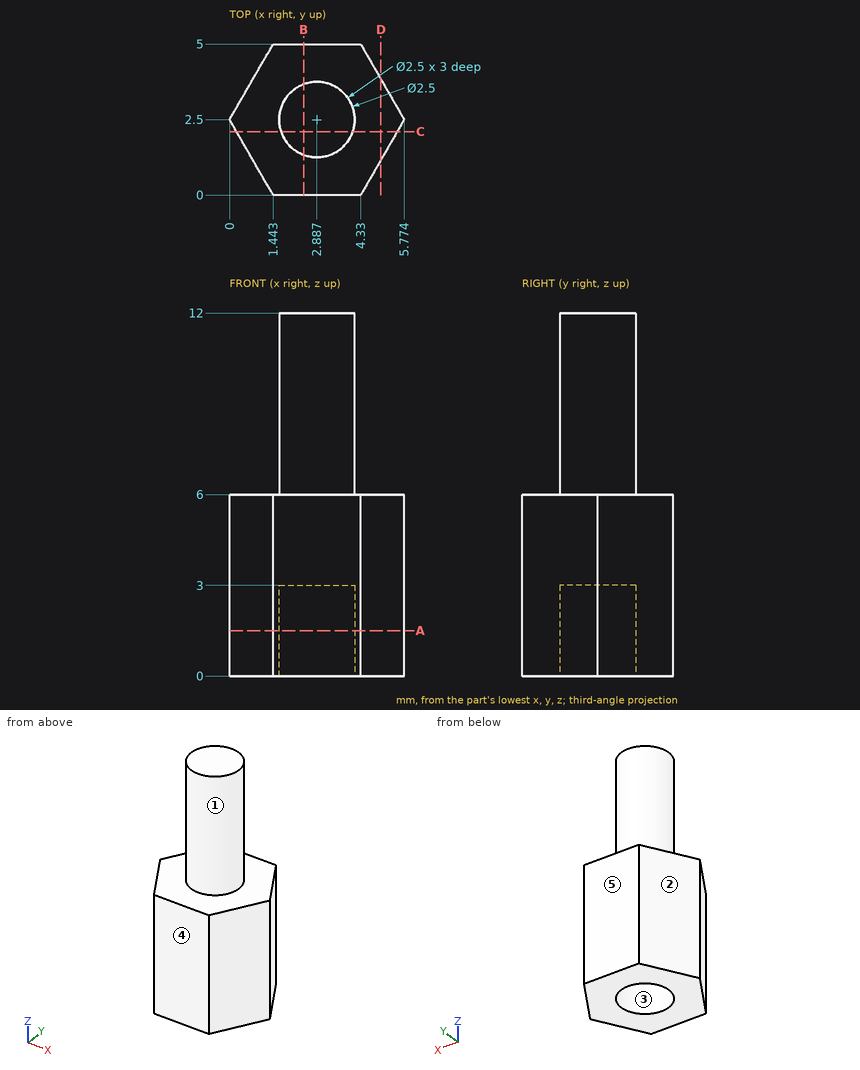
Geometry check sheet. Reference: drawing and pictorial views, mm from the part's lowest x, y, z. A direction names the side the tool comes from. Coordinates: 2 decimals unless noted, no trailing zeros. Order: outer loops, then holes, each group sorted by start corner. A loop starts at its lowest first (then second) coordinate and runs counter-clockwise, first axis right, second up. Notation, with made-up numbers: M -30.75,78 L 17.25,78 A28 ccw 17.25,110 Z; hole C 79,87.25 d5. An arc over 180 degrees is marked long. Write each question's results on one line, items separated by ' | '. Start each with the question number.
1. Material ranges on probe 1 along Z at (x, y) = (1.4, 4); probe 2 along Y at (x, z) = (2.9, 10.5); probe 3 along X at (y, z) = (2.35, 1.25) (1 decimal), recorded low to high.
2. Cross-section at B-B on x = 2.45. Record the cut outline in (y, z).
3. Mould release check, pull along Y, two halves, no side actions. Record for the marked faces 3, 4 and 5: +Y half, -Y half, draft (parallel to the pull), parting line (faces both ways), or undercut.
4. Access from +Z, -Z, +X, -X, +Y, -Y to the whole of each face (thin tool, end or side, straight path). Record for the marked faces 1 and 2.
5. Cross-section at D-D on x = 5. Record the cut outline in (y, z), and give its area (3 significant figures).
6. Go/stop test with flat-tipped pins: P1, Ø1.5, axis at y = 3.5, z = 8.5, coming from the +X side; P2, Ø3, axis at x = 3.5, y = 2.5, coming from the -Z side. Record where each tip stops, or that it passes through.
7. Cross-section at A-A on z = 1.5. Record the cut outline in (x, y).
8. Cross-section at C-C on y = 2.1. Record the cut outline in (x, z).
Checks:
1) probe 1: z = 0 to 6 | probe 2: y = 1.25 to 3.75 | probe 3: x = 0.1 to 1.6, 4.1 to 5.7
2) outline: M 0,0 L 1.33,0 L 1.33,3 L 3.67,3 L 3.67,0 L 5,0 L 5,6 L 3.67,6 L 3.67,12 L 1.33,12 L 1.33,6 L 0,6 Z
3) face 3: undercut | face 4: -Y half | face 5: +Y half
4) face 1: +Z | face 2: +Z, -Z, -X, +Y
5) outline: M 1.16,0 L 3.84,0 L 3.84,6 L 1.16,6 Z | area: 16.1 mm²
6) P1: stops at x = 4.11 | P2: stops at z = 0
7) outline: M 0,2.5 L 1.44,0 L 4.33,0 L 5.77,2.5 L 4.33,5 L 1.44,5 Z; hole C 2.89,2.5 d2.5
8) outline: M 0.23,0 L 1.7,0 L 1.7,3 L 4.07,3 L 4.07,0 L 5.54,0 L 5.54,6 L 4.07,6 L 4.07,12 L 1.7,12 L 1.7,6 L 0.23,6 Z
